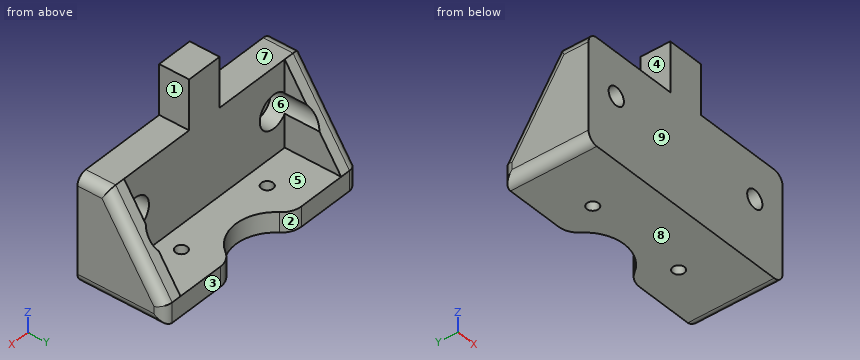
```python
from build123d import *

# Parameters (mm, degrees)
BOSS_EXTRUDE1_DEPTH = 9
BOSS_EXTRUDE2_DEPTH = 6
BOSS_EXTRUDE3_DEPTH = 6
SKETCH4_R           = 2.75
CUT_EXTRUDE1_DEPTH  = 50.749371855
CUT_EXTRUDE2_START  = -5
SKETCH5_R           = 5
CUT_EXTRUDE2_DEPTH  = 55.749371855
SKETCH6_R           = 1.75
CUT_EXTRUDE3_DEPTH  = 60.84981203
FILLET1_R           = 3


with BuildPart() as part:
    # Sketch1 → Boss-Extrude1 (new body)
    with BuildSketch(Plane(origin=(0, 0, 0), x_dir=(1, 0, 0), z_dir=(0, 1, 0))):
        Polygon((5.5, -16), (35, -16), (35, 16), (-35, 16), (-35, -16), (-5.5, -16), (-5.5, -31), (5.5, -31), align=None)
    extrude(amount=BOSS_EXTRUDE1_DEPTH)

    # Sketch2 → Boss-Extrude2 (add)
    with BuildSketch(Plane(origin=(0, 0, -16), x_dir=(-1, 0, 0), z_dir=(0, 0, -1))):
        with BuildLine():
            Line((-35, 9), (35, 9))
            Line((35, 9), (35, 26))
            Line((35, 26), (14.620191517, 26))
            ThreePointArc((14.620191517, 26), (11.88157873, 25.338539126), (9.746794345, 23.5))
            ThreePointArc((9.746794345, 23.5), (0, 18.5), (-9.746794345, 23.5))
            ThreePointArc((-9.746794345, 23.5), (-11.88157873, 25.338539126), (-14.620191517, 26))
            Line((-14.620191517, 26), (-35, 26))
            Line((-35, 26), (-35, 9))
        make_face()
    extrude(amount=-BOSS_EXTRUDE2_DEPTH)

    # Sketch3 → Boss-Extrude3 (add)
    with BuildSketch(Plane(origin=(35, 0, 0), x_dir=(0, 0, -1), z_dir=(1, 0, 0))):
        Polygon((-16, 9), (10, 26), (10, 9), align=None)
    boss_extrude3 = extrude(amount=-BOSS_EXTRUDE3_DEPTH)

    # Sketch4 → Cut-Extrude1 (cut, through all)
    with BuildSketch(Plane(origin=(0, 9, 0), x_dir=(1, 0, 0), z_dir=(0, 1, 0))):
        with Locations(Location((25, -3, 0), (0, 0, 270))):
            Circle(SKETCH4_R)
    cut_extrude1 = extrude(amount=-CUT_EXTRUDE1_DEPTH, mode=Mode.SUBTRACT)

    # Sketch5 → Cut-Extrude2 (cut)
    with BuildSketch(Plane(origin=(0, 9, 0), x_dir=(1, 0, 0), z_dir=(0, 1, 0)).offset(CUT_EXTRUDE2_START)):
        with Locations(Location((25, -3, 0), (0, 0, 36.869897646))):
            Circle(SKETCH5_R)
    cut_extrude2 = extrude(amount=CUT_EXTRUDE2_DEPTH, mode=Mode.SUBTRACT)

    # Sketch6 → Cut-Extrude3 (cut, through all)
    with BuildSketch(Plane.XY.offset(-10)):
        with Locations((15.5, 15)):
            Circle(SKETCH6_R)
    cut_extrude3 = extrude(amount=-CUT_EXTRUDE3_DEPTH, mode=Mode.SUBTRACT)

    # Mirror1: Boss-Extrude3, Cut-Extrude1, Cut-Extrude2, Cut-Extrude3 across plane
    add(boss_extrude3.mirror(Plane(origin=(0, 0, 0), x_dir=(0, 0, 1), z_dir=(1, 0, 0))))
    add(cut_extrude1.mirror(Plane(origin=(0, 0, 0), x_dir=(0, 0, 1), z_dir=(1, 0, 0))), mode=Mode.SUBTRACT)
    add(cut_extrude2.mirror(Plane(origin=(0, 0, 0), x_dir=(0, 0, 1), z_dir=(1, 0, 0))), mode=Mode.SUBTRACT)
    add(cut_extrude3.mirror(Plane(origin=(0, 0, 0), x_dir=(0, 0, 1), z_dir=(1, 0, 0))), mode=Mode.SUBTRACT)

    # Fillet1
    fillet1_edges = [part.edges().sort_by_distance(p)[0] for p in [
        (35, 4.5, 16),
        (-35, 4.5, 16),
        (-35, 13, -16),
        (35, 13, -16),
        (35, 26, -13),
        (-35, 26, -13),
        (35, 17.5, 3),
        (-35, 17.5, 3),
    ]]
    fillet(fillet1_edges, radius=FILLET1_R)


solid = part.part
```
The listing builds one solid part. Answer for the finished solid, in the listing's coordinates (mm). Face numbers are marked on the shaded views. A direction names the side the tool comes from. Give positions to 0.01 mm unless a question says otherwise; leave off trailing zeros. Loops run counter-clockwise (first coordinate to the right, second up) from the corner with the lowest first, then second, coordinate; pieces in that order, holes last. Notation, with made-up numbers: (-4.5, 46) - (2.5, 46) arc R14 ccw to (2.5, 56) - close; hole circle Ø2 at (36, -2). An arc over 180 degrees is marked (long way). Return JSON: item names as keys, results as strings. Group by question number.
1. Determine the mould class of the marked faces 6, 7, 8 and 9 for opening direction Z: pulls with the +Z half, pulls with the -Z half, needs draft (parallel to the pull), parting line crosses it, or undercut.
2. Find section D-D (x = -18). Write down the section's boundary in (y, z), then the cut area to 3 significant figures.
3. Find section A-A (x = 15.5). Write down the section's boundary in (y, z), then the cut area to 3 significant figures.
4. Find section B-B (z = 26). Write down the section's boundary in (x, y).
5. Find section C-C (x = 25). Write down the section's boundary in (y, z).
6. Given pin 1 Ø1 at (y, z) = (7, 18) entering from +X; pin 2 Ø20.5 at (x, z) = (-12.5, 14) entering from +Y; pin 3 Ø3.5 at (y, z) = (13, 9) entering from +X; pin 4 Ø10 at (y, z) = (4, 17) entering from -X, each flat-ended and moving along its own axis, determine where each tip first touches the part or whether it passes through.
7. Straight lines are drawn through the part: line 1 (Y direction, x = 15.5, z = -13.1); line 2 (Y direction, x = -1.5, z = 29.5); line 3 (Z direction, x = 25, y = 16.25). For each, find the intervals that lie inside material, in ascending order. Write a range as [from, to].
8. Which of the six approach directions +Z, -Z, +X, -X, +Y, -Y give full straight-line access (tool end or side, diameter ignored) to the marked faces 1, 2, 3, 4 and 5?
Verdict:
{
 "1": {"face 6": "undercut", "face 7": "pulls with the +Z half", "face 8": "pulls with the -Z half", "face 9": "needs draft"},
 "2": {"outline": "(0, -16) - (26, -16) - (26, -10) - (9, -10) - (9, 16) - (0, 16) - close", "area": "390 mm^2"},
 "3": {"outline": "(0, -16) - (13.25, -16) - (13.25, -10) - (9, -10) - (9, 16) - (0, 16) - close; (16.75, -16) - (26, -16) - (26, -10) - (16.75, -10) - close", "area": "369 mm^2"},
 "4": {"outline": "(-5.5, 0) - (5.5, 0) - (5.5, 9) - (-5.5, 9) - close"},
 "5": {"outline": "(0, -16) - (26, -16) - (26, -10) - (9, -10) - (9, -2) - (4, -2) - (4, 0.25) - (0, 0.25) - close; (0, 5.75) - (4, 5.75) - (4, 8) - (9, 8) - (9, 16) - (0, 16) - close"},
 "6": {"pin 1": "stops at x = 5.5", "pin 2": "stops at y = 9", "pin 3": "stops at x = 34.9", "pin 4": "stops at x = -35"},
 "7": {"line 1": "y = [0, 13.25], [16.75, 26]", "line 2": "y = [0, 9]", "line 3": "z = [-16, -10]"},
 "8": {"face 1": "+Z, +X, +Y, -Y", "face 2": "+Z, -Z, +Y", "face 3": "+Z, -Z, +X, -X, +Y", "face 4": "+Z, -X, +Y, -Y", "face 5": "+Z, +Y"}
}
